```python
from build123d import *

# Parameters (mm, degrees)
EXTRUDE_1_DEPTH     = 25
SKETCH_2_R          = 12.5
CUT_EXTRUDE_1_DEPTH = 11
SKETCH_3_R          = 4.5
CUT_EXTRUDE_2_DEPTH = 15
SKETCH_5_R          = 8
CUT_EXTRUDE_3_DEPTH = 9
SKETCH_6_R          = 4
CUT_EXTRUDE_4_DEPTH = 50


with BuildPart() as part:
    # 草图1 → 凸台-拉伸1 (new body)
    with BuildSketch(Plane(origin=(0, 0, 0), x_dir=(1, 0, 0), z_dir=(0, 1, 0))):
        with BuildLine():
            Line((-50, -125), (45, -125))
            ThreePointArc((45, -125), (48.535533906, -123.535533906), (50, -120))
            Line((50, -120), (50, 120))
            ThreePointArc((50, 120), (48.535533906, 123.535533906), (45, 125))
            Line((45, 125), (-50, 125))
            Line((-50, 125), (-50, -125))
        make_face()
    extrude(amount=EXTRUDE_1_DEPTH)

    # 草图2 → 切除-拉伸1 (cut)
    with BuildSketch(Plane(origin=(0, 25, 0), x_dir=(1, 0, 0), z_dir=(0, 1, 0))):
        with Locations(Location((-17.5, 90, 0), (0, 0, 270))):
            Circle(SKETCH_2_R)
        with Locations(Location((-17.5, -90, 0), (0, 0, 270))):
            Circle(SKETCH_2_R)
    extrude(amount=-CUT_EXTRUDE_1_DEPTH, mode=Mode.SUBTRACT)

    # 草图3 → 切除-拉伸2 (cut)
    with BuildSketch(Plane(origin=(0, 14, 0), x_dir=(1, 0, 0), z_dir=(0, 1, 0))):
        with Locations(Location((-17.5, 90, 0), (0, 0, 270))):
            Circle(SKETCH_3_R)
        with Locations(Location((-17.5, -90, 0), (0, 0, 270))):
            Circle(SKETCH_3_R)
    extrude(amount=-CUT_EXTRUDE_2_DEPTH, mode=Mode.SUBTRACT)

    # 草图5 → 切除-拉伸3 (cut)
    with BuildSketch(Plane.XZ):
        with Locations(Location((-17.5, 90, 0), (0, 0, 270))):
            Circle(SKETCH_5_R)
        with Locations(Location((-17.5, -90, 0), (0, 0, 270))):
            Circle(SKETCH_5_R)
    extrude(amount=-CUT_EXTRUDE_3_DEPTH, mode=Mode.SUBTRACT)

    # 草图6 → 切除-拉伸4 (cut)
    with BuildSketch(Plane.ZY.offset(50)):
        with Locations((112, 12.5)):
            Circle(SKETCH_6_R)
        with Locations(Location((-112, 12.5, 0), (0, 0, 180))):
            Circle(SKETCH_6_R)
    extrude(amount=-CUT_EXTRUDE_4_DEPTH, mode=Mode.SUBTRACT)


solid = part.part
```
CAD build for the part. Positions are in the model's coordinates, mm. A direction names the side the tool comes from. Coordinates: 2 decimals unless noted, no trailing zeros. Write each loop counter-clockwise with the first axis right and the second up, starting at its lowest first coordinate (ties: lowest second). Pieces come first, ordered by that corner, then holes.
(1) 3-axis set-ups, long thin cutter, end or side, ignore diameter. For faces 5 (the face through (-25.35, 12.324, -108.004)), 6 (the face through (-22.368, 4.437, 96.349)), 7 (the face through (-23, 14, 90)): which of +Z, -Z, +X, -X, +Y, -Y reach the whole face in a straight line?
(2) Cut at A-A, the plane z = 90. List the corners of the cut face in (x, y), and give its area (3 significant figures).
(3) Drill centre lines: probe 1 along Z at (x, y) = (-21, 19); probe 2 along X at (y, z) = (17.5, -90); probe 3 along Z at (x, y) = (-39, 13.75). Where is each one in solid material? Low to high.
(4) Flat gauge pins, fed straight in: pin 1 (6.5 mm diameter, centred on y = 12.5, z = 112, fed in from -X); pin 2 (8 mm diameter, centred on x = -17, z = -87, fed in from -Y); pin 3 (12.5 mm diameter, centred on x = -15, z = 95, fed in from +Y). Where does each tip first touch, or does it go through?
(5) Two-plate mould, pull along Z, no slides. Class faces 1 (the face through (-2, 12, -125)), 2 (the face through (-3, 12, 125)), 3 (the face through (-50, 12, -2)), 4 (the face through (0, 13, 112)): +Z half, -Z half, draft (parallel to the pull), parting line (faces both ways), or undercut.
(6) Cut at C-C, the plane y = 5. List the corners of the cut face in (x, z), and give its area (3 significant figures).
(7) Cut at B-B, the plane x = -17.5. Count the separate pieces of the cut face and the enclosed holes in it, and give its area (3 significant figures).
(8) Cut at D-D, the plane z = -112. List the corners of the cut face in (x, y), and give its area (3 significant figures).
Geometry says:
1. face 5: -X
1. face 6: -Y
1. face 7: +Y
2. outline: (-50, 0) - (-25.5, 0) - (-25.5, 9) - (-22, 9) - (-22, 14) - (-30, 14) - (-30, 25) - (-50, 25) - close; (-13, 9) - (-9.5, 9) - (-9.5, 0) - (50, 0) - (50, 25) - (-5, 25) - (-5, 14) - (-13, 14) - close
2. area: 2,040 mm2
3. probe 1: z = -125 to -102, -78 to 78, 102 to 125
3. probe 2: x = -50 to -30, -5 to 50
3. probe 3: z = -125 to -115.8, -108.2 to 108.2, 115.8 to 125
4. pin 1: stops at x = 0
4. pin 2: stops at y = 9
4. pin 3: stops at y = 14
5. face 1: -Z half
5. face 2: +Z half
5. face 3: draft
5. face 4: undercut
6. outline: (-50, -125) - (45, -125) arc R5 ccw to (50, -120) - (50, 120) arc R5 ccw to (45, 125) - (-50, 125) - close; hole circle Ø16 at (-17.5, -90); hole circle Ø16 at (-17.5, 90)
6. area: 24,600 mm2
7. separate pieces: 3
7. enclosed holes: 2
7. area: 5,220 mm2
8. outline: (-50, 0) - (50, 0) - (50, 25) - (-50, 25) - (-50, 16.5) - (0, 16.5) - (0, 8.5) - (-50, 8.5) - close
8. area: 2,100 mm2
